from build123d import *

# Parameters (mm, degrees)
SKETCH1_W            = 40
SKETCH1_H            = 50
BOSS_EXTRUDE1_DEPTH  = 5
SKETCH3_W            = 5
SKETCH3_H            = 5
BOSS_EXTRUDE5_DEPTH  = 20
SKETCH3_3_W          = 15
SKETCH3_3_H          = 5
BOSS_EXTRUDE6_DEPTH  = 10
CUT_EXTRUDE3_DEPTH   = 4
BOSS_EXTRUDE9_START  = 3
BOSS_EXTRUDE9_DEPTH  = 3
SKETCH12_W           = 5
SKETCH12_H           = 5
BOSS_EXTRUDE10_DEPTH = 5
SKETCH13_R           = 1.5
CUT_EXTRUDE4_DEPTH   = 5
SKETCH16_W           = 5
SKETCH16_H           = 2.5
BOSS_EXTRUDE13_DEPTH = 5
BOSS_EXTRUDE14_DEPTH = 10
SKETCH17_R           = 1.5
CUT_EXTRUDE6_DEPTH   = 2.5


with BuildPart() as part:
    # Sketch1 → Boss-Extrude1 (new body)
    with BuildSketch(Plane(origin=(0, 0, 0), x_dir=(1, 0, 0), z_dir=(0, 1, 0))):
        Rectangle(SKETCH1_W, SKETCH1_H)
    extrude(amount=BOSS_EXTRUDE1_DEPTH)

    # Sketch3 → Boss-Extrude5 (add)
    with BuildSketch(Plane(origin=(0, 5, 0), x_dir=(1, 0, 0), z_dir=(0, 1, 0))):
        with Locations((17.5, -22.5)):
            Rectangle(SKETCH3_W, SKETCH3_H)
        with Locations((9.5, 22.5)):
            Rectangle(SKETCH3_W, SKETCH3_H)
    extrude(amount=BOSS_EXTRUDE5_DEPTH)

    # Sketch3_3 → Boss-Extrude6 (add)
    with BuildSketch(Plane(origin=(0, 5, 0), x_dir=(1, 0, 0), z_dir=(0, 1, 0))):
        with Locations((-0.5, 22.5)):
            Rectangle(SKETCH3_3_W, SKETCH3_3_H)
        Polygon((-16, -20), (-16, 25), (-20, 25), (-20, -25), (7, -25), (7, -20), align=None)
    extrude(amount=BOSS_EXTRUDE6_DEPTH)

    # Sketch8 → Cut-Extrude3 (cut)
    with BuildSketch(Plane.ZY.offset(20)):
        with BuildLine():
            Line((1, 15), (-21, 15))
            ThreePointArc((-21, 15), (-10, 4), (1, 15))
        make_face()
    extrude(amount=-CUT_EXTRUDE3_DEPTH, mode=Mode.SUBTRACT)

    # Sketch10 → Boss-Extrude9 (add)
    with BuildSketch(Plane.ZY.offset(20).offset(BOSS_EXTRUDE9_START)):
        with BuildLine():
            Line((1, 15), (4, 15))
            Line((4, 15), (4, 0))
            Line((4, 0), (-24, 0))
            Line((-24, 0), (-24, 15))
            Line((-24, 15), (-21, 15))
            ThreePointArc((-21, 15), (-10, 4), (1, 15))
        make_face()
    extrude(amount=-BOSS_EXTRUDE9_DEPTH)

    # Sketch12 → Boss-Extrude10 (add)
    with BuildSketch(Plane(origin=(0, 0, -25), x_dir=(-1, 0, 0), z_dir=(0, 0, -1))):
        with Locations((0, 12.5)):
            Rectangle(SKETCH12_W, SKETCH12_H)
    extrude(amount=BOSS_EXTRUDE10_DEPTH)

    # Sketch13 → Cut-Extrude4 (cut)
    with BuildSketch(Plane.XZ.offset(-10)):
        with Locations(Location((0, -27.5, 0), (0, 0, 270))):
            Circle(SKETCH13_R)
    extrude(amount=-CUT_EXTRUDE4_DEPTH, mode=Mode.SUBTRACT)

    # Sketch16 → Boss-Extrude13 (add)
    with BuildSketch(Plane.XY.offset(25)):
        with Locations((-10, 11.25)):
            Rectangle(SKETCH16_W, SKETCH16_H)
    extrude(amount=BOSS_EXTRUDE13_DEPTH)

    # Sketch16_3 → Boss-Extrude14 (add)
    with BuildSketch(Plane.XY.offset(25)):
        Polygon((-7.5, 5), (7, 5), (7, 12.5), (-7.5, 12.5), (-7.5, 10), align=None)
    extrude(amount=BOSS_EXTRUDE14_DEPTH)

    # Sketch17 → Cut-Extrude6 (cut)
    with BuildSketch(Plane.XZ.offset(-10)):
        with Locations((-10, 27.5)):
            Circle(SKETCH17_R)
    extrude(amount=-CUT_EXTRUDE6_DEPTH, mode=Mode.SUBTRACT)


solid = part.part
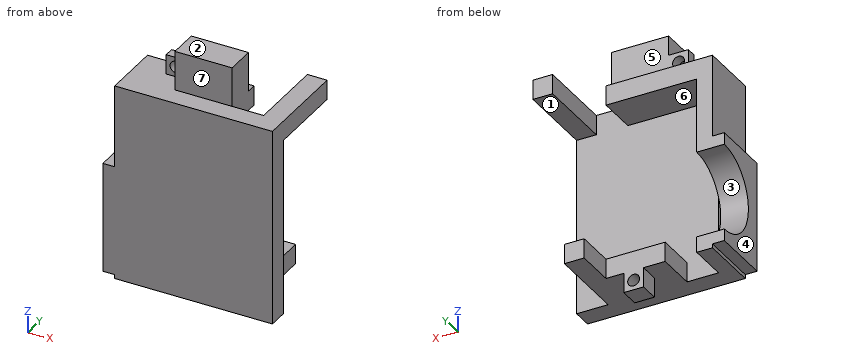
Verification items for the finished model (mm, model axes). Face numbers are marked on the shaded views. A direction names the side the tool comes from. Coordinates: 2 decimals unless noted, no trailing zeros. Write each loop counter-clockwise with the first axis right and the second up, starting at its lowest first coordinate (ties: lowest second). Pieces come first, ordered by that corner, then holes. Notation, with made-up numbers: (30, 73.25) - (38, 73.25) arc R21 cw to (38, 82.25) - close; hole circle Ø3 at (-12, -31.5). An arc over 180 degrees is marked (long way). Answer as a JSON object with one key per item and string values.
(1) Mould release check, pull along Z, two halves, no side actions. Record for the marked faces 1, 2, 3 and 4: pulls with the +Z half, pulls with the -Z half, needs draft (parallel to the pull), parting line crosses it, or undercut.
Report:
{"face 1": "pulls with the -Z half", "face 2": "pulls with the +Z half", "face 3": "undercut", "face 4": "needs draft"}
(2) Thickness scan on line 1 along X through (y, z) = (12.25, -27.5); line 2 along Z through (x, y) = (-7, 10); line 3 along Z through (x, y) = (-13, 2). Record the ranges inside material, lowest first.
Report:
{"line 1": "-2.5 to -1.5, 1.5 to 2.5", "line 2": "-25 to -20, 20 to 35", "line 3": "-25 to 25"}
(3) Cross-section at A-A on x = -10. Record the cut outline in (y, z), plus the area to 3 significant figures.
Report:
{"outline": "(0, -25) - (5, -25) - (5, 20) - (15, 20) - (15, 25) - (12.5, 25) - (12.5, 26) - (10, 26) - (10, 25) - (0, 25) - close; (10, 29) - (12.5, 29) - (12.5, 30) - (10, 30) - close", "area": "305 mm^2"}
(4) Cross-section at D-D on x = 0. Record the cut outline in (y, z).
Report:
{"outline": "(0, -25) - (10, -25) - (10, -26) - (15, -26) - (15, -20) - (5, -20) - (5, 20) - (15, 20) - (15, 25) - (12.5, 25) - (12.5, 35) - (5, 35) - (5, 25) - (0, 25) - close; (10, -30) - (15, -30) - (15, -29) - (10, -29) - close"}
(5) Gauge pin test, flat ends, axial feed: pin 1 Ø6 at (x, y) = (10.5, 17) entering from -Z; pin 2 Ø0.5 at (y, z) = (10, -24.5) entering from -X; pin 3 Ø2.5 at (x, z) = (0, -27.5) entering from -Y; pin 4 Ø6 at (x, z) = (-9, 27) entering from +Y. Record the tip position at first contact, or that the pin passes through.
Report:
{"pin 1": "z = -25", "pin 2": "x = -20", "pin 3": "through", "pin 4": "y = 15"}
(6) Cross-section at B-B on y = 17.5. Record the cut outline in (x, z), plus the area to 3 significant figures.
Report:
{"outline": "(7, -25) - (12, -25) - (12, -20) - (7, -20) - close; (15, 20) - (20, 20) - (20, 25) - (15, 25) - close", "area": "50.0 mm^2"}
(7) Tool access check on the marked faces 5, 6 and 7. Record the directions out of +Z, -Z, +X, -X, +Y, -Y that give a thin tool (end or side, any length) a straight path to the whole face; none if there is none.
Report:
{"face 5": "+Z, +X, -X, +Y", "face 6": "+X, +Y", "face 7": "+Z, +X, -X, -Y"}
(8) Cross-section at C-C on z = -27.5. Record the cut outline in (x, y), plus the area to 3 significant figures.
Report:
{"outline": "(-2.5, 10) - (-1.5, 10) - (-1.5, 15) - (-2.5, 15) - close; (1.5, 10) - (2.5, 10) - (2.5, 15) - (1.5, 15) - close", "area": "10.0 mm^2"}
